The listing builds one solid part. Answer for the finished solid, in the listing's coordinates (mm). A direction names the side the tool comes from. Round coordinates to 2 decimals unless told otherwise and drop trailing zeros. Write each loop counter-clockwise with the first axis right and the second up, starting at its lowest first coordinate (ties: lowest second). Pieces come first, ordered by that corner, then holes.
Item 1: For a pull along Y with two mould halves and no side action, classify faces 1 (the face through (6.35, 148, 10)), 2 (the face through (3, 115, 14.05)), 3 (the face through (3, 0, 10)) as +Y half, -Y half, draft (parallel to the pull), parting line (faces both ways), or undercut.
Item 2: This flat-tipped pin is pushed along its axis until it touches: pin 1 (3 mm diameter, centred on x = 3.5, y = 39.5, fed in from -Z). Where does it stop, or does it pass through?
Item 3: Find the intervals of material crossed by probe 1 along Z at (x, y) = (5.5, 15); probe 2 along X at (y, z) = (7.5, 10.5); probe 3 along Z at (x, y) = (0.75, 47.5), in increasing order.
Item 4: Find section A-A on y = 176.5. Give the vertices of the cut face in (x, z).
Item 5: A tool of negligible diameter and unlimited length cuts with its end or side. For faces 4 (the face through (0, 148, 10)), 5 (the face through (3, 258, 5)), from which of +Z, -Z, +X, -X, +Y, -Y can it reach the whole face along a straight path? Write none if from no direction.
Autodesk Inventor part; units mm, degrees
ref_plane "YZ Plane" through (0, 0, 0) normal (1, 0, 0) x (0, 1, 0)
ref_plane "XZ Plane" through (0, 0, 0) normal (0, 1, 0) x (-1, 0, 0)
ref_plane "XY Plane" through (0, 0, 0) normal (0, 0, 1) x (1, 0, 0)
sketch "Sketch1" plane through (0, 0, 0) normal (1, 0, 0) x (0, 1, 0)
  line L0 (0, 0) -> (300, 0)
  line L1 (300, 0) -> (300, 19.05)
  line L2 (300, 19.05) -> (0, 19.05)
  line L3 (0, 19.05) -> (0, 0)
  dimension "d0" = 300
  dimension "d1" = 19.05
extrude "Extrusion1" add sketch "Sketch1" along normal blind 6.35
sketch "Sketch2" plane through (6.35, 0, 0) normal (1, 0, 0) x (0, 0, -1)
  line L0 (0, 300) -> (-19.05, 300)
  line L1 (-19.05, 300) -> (-19.05, 0)
  line L2 (-19.05, 0) -> (0, 0)
  point P0 (-9.525, 285)
  point P1 (-9.525, 150)
  point P2 (-9.525, 15)
  dimension "d4" = 15
  dimension "d5" = 19.05
  dimension "d6" = 9.525
  dimension "d7" = 15
  dimension "d8" = 9.525
  dimension "d9" = 9.525
  dimension "d10" = 150
hole "Hole1" at (6.35, 285, 9.525) at (6.35, 150, 9.525) at (6.35, 15, 9.525) direction (-1, 0, 0) diameter 3.302 end through all
sketch "Sketch5" plane through (6.35, 0, 0) normal (1, 0, 0) x (0, 0, -1)
  line L0 (-14.05, 270) -> (-5, 270)
  line L1 (-5, 270) -> (-5, 245)
  line L2 (-5, 245) -> (-14.05, 245)
  line L3 (-14.05, 245) -> (-14.05, 270)
  line L4 (-14.05, 205) -> (-5, 205)
  line L5 (-5, 205) -> (-5, 165)
  line L6 (-5, 165) -> (-14.05, 165)
  line L7 (-14.05, 165) -> (-14.05, 205)
  line L8 (-14.05, 135) -> (-5, 135)
  line L9 (-5, 135) -> (-5, 95)
  line L10 (-5, 95) -> (-14.05, 95)
  line L11 (-14.05, 95) -> (-14.05, 135)
  line L12 (-14.05, 55) -> (-5, 55)
  line L13 (-5, 55) -> (-5, 30)
  line L14 (-5, 30) -> (-14.05, 30)
  line L15 (-14.05, 30) -> (-14.05, 55)
  line L16 (0, 0) -> (0, 300)
  line L17 (-19.05, 300) -> (-19.05, 0)
  line L18 (0, 300) -> (-19.05, 300)
  line L19 (-19.05, 0) -> (0, 0)
  dimension "d44" = 5
  dimension "d45" = 5
  dimension "d46" = 30
  dimension "d47" = 30
  dimension "d48" = 55
  dimension "d49" = 95
  dimension "d50" = 135
  dimension "d51" = 55
  dimension "d52" = 95
  dimension "d53" = 135
extrude "Extrusion2" cut sketch "Sketch5" against normal through all contours L0 L1 L2 L3 | L4 L5 L6 L7 | L8 L9 L10 L11 | L12 L13 L14 L15
fillet "Fillet1" radius 3.175 1 edges at (3.175, 270, 5)
fillet "Fillet2" radius 3.175 1 edges at (3.175, 270, 14.05)
fillet "Fillet3" radius 3.175 1 edges at (3.175, 245, 5)
fillet "Fillet4" radius 3.175 1 edges at (3.175, 245, 14.05)
fillet "Fillet5" radius 3.175 1 edges at (3.175, 205, 5)
fillet "Fillet6" radius 3.175 1 edges at (3.175, 205, 14.05)
fillet "Fillet7" radius 3.175 1 edges at (3.175, 165, 5)
fillet "Fillet8" radius 3.175 1 edges at (3.175, 165, 14.05)
fillet "Fillet9" radius 3.175 1 edges at (3.175, 95, 5)
fillet "Fillet10" radius 3.175 1 edges at (3.175, 135, 5)
fillet "Fillet11" radius 3.175 1 edges at (3.175, 135, 14.05)
fillet "Fillet12" radius 3.175 1 edges at (3.175, 95, 14.05)
fillet "Fillet13" radius 3.175 1 edges at (3.175, 55, 5)
fillet "Fillet14" radius 3.175 1 edges at (3.175, 55, 14.05)
fillet "Fillet15" radius 3.175 1 edges at (3.175, 30, 14.05)
fillet "Fillet16" radius 3.175 1 edges at (3.175, 30, 5)
sketch "Sketch7" plane through (0, 0, 0) normal (0, 0, -1) x (-1, 0, 0)
  line L0 (0, 300) -> (-6.35, 300)
  line L1 (0, 0) -> (-6.35, 0)
  line L2 (-6.35, 0) -> (-6.35, 300)
  point P0 (-3.175, 7.5)
  point P1 (-3.175, 22.5)
  point P2 (-3.175, 142.5)
  point P3 (-3.175, 157.5)
  point P4 (-3.175, 277.5)
  point P5 (-3.175, 292.5)
  dimension "d72" = 7.5
  dimension "d73" = 22.5
  dimension "d74" = 142.5
  dimension "d78" = 7.5
  dimension "d79" = 22.5
  dimension "d82" = 142.5
  dimension "d83" = 6.35
  dimension "d84" = 3.175
  dimension "d85" = 3.175
  dimension "d88" = 3.175
  dimension "d89" = 3.175
  dimension "d92" = 3.175
  dimension "d93" = 3.175
hole "Hole3" at (3.175, 7.5, 0) at (3.175, 22.5, 0) at (3.175, 142.5, 0) at (3.175, 157.5, 0) at (3.175, 277.5, 0) at (3.175, 292.5, 0) direction (0, 0, 1) diameter 2.6416 end through all
equation "\"d45\" = d44"
equation "\"d47\" = d46"
equation "\"d51\" = d48"
equation "\"d52\" = d49"
equation "\"d53\" = d50"
equation "\"d87\" = d84"
equation "\"d91\" = d89"
properties part number "slides"
Check values:
1. face 1: draft
1. face 2: undercut
1. face 3: -Y half
2. pin 1: stops at z = 0
3. probe 1: z = 0 to 7.87, 11.18 to 19.05
3. probe 2: x = 0 to 1.85, 4.5 to 6.35
3. probe 3: z = 0 to 5, 14.05 to 19.05
4. outline: (0, 0) - (6.35, 0) - (6.35, 5) - (0, 5) - close; (0, 14.05) - (6.35, 14.05) - (6.35, 19.05) - (0, 19.05) - close
5. face 4: +Z, -Z, -X, +Y, -Y
5. face 5: +X, -X
